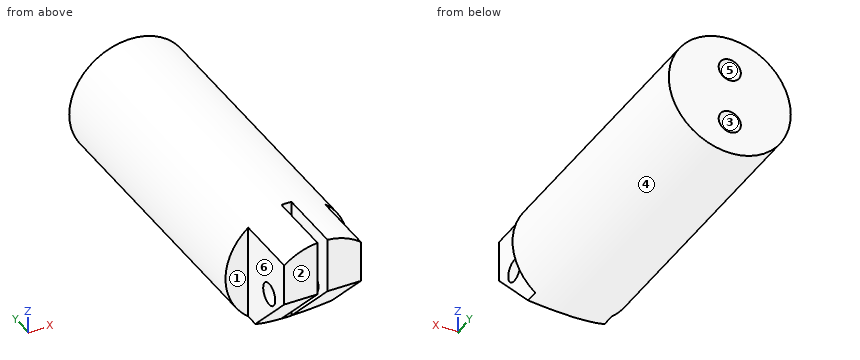
Autodesk Inventor part; units mm, degrees
ref_plane "YZ Plane" through (0, 0, 0) normal (1, 0, 0) x (0, 1, 0)
ref_plane "XZ Plane" through (0, 0, 0) normal (0, 1, 0) x (-1, 0, 0)
ref_plane "XY Plane" through (0, 0, 0) normal (0, 0, 1) x (1, 0, 0)
sketch "Sketch1" plane through (0, 0, 0) normal (0, 1, 0) x (-1, 0, 0)
  circle A0 centre (0, 0) radius 5.5
  dimension "d0" = 11
extrude "Extrusion1" add sketch "Sketch1" along normal blind 26
sketch "Sketch6" plane through (0, 0, 0) normal (0, -1, 0) x (1, 0, 0)
  circle A0 centre (0, 0) radius 5.5
  line L0 (3.45, 0) -> (3.45, -4.2834)
  line L1 (0.45, 0) -> (0.45, -5.4816)
  line L2 (3.45, -5.4816) -> (3.45, -4.2834)
  line L3 (3.45, -5.4816) -> (0.45, -5.4816)
  line L4 (0.45, 0) -> (0.45, 5.4816)
  line L5 (3.45, 5.3243) -> (3.45, 0)
  line L6 (3.45, 5.3243) -> (0.45, 5.4816)
  line L7 (0, -5.5) -> (0, 5.5)
  line L8 (-3.45, 0) -> (-3.45, -4.2834)
  line L9 (-0.45, 0) -> (-0.45, -5.4816)
  line L10 (-3.45, -5.4816) -> (-3.45, -4.2834)
  line L11 (-3.45, -5.4816) -> (-0.45, -5.4816)
  line L12 (-0.45, 0) -> (-0.45, 5.4816)
  line L13 (-3.45, 5.3243) -> (-3.45, 0)
  line L14 (-3.45, 5.3243) -> (-0.45, 5.4816)
  point P0 (-3.45, 4.2834)
  point P1 (3.45, 4.2834)
  dimension "d20" = 3
  dimension "d21" = 3
  dimension "d22" = 0.45
  dimension "d23" = 2.05
  dimension "d24" = 2.05
extrude "Extrusion5" add sketch "Sketch6" along normal blind 6 contours A0 L5 L0 L1 L4 | L12 L9 A0 L8 L13
sketch "Sketch8" plane through (0, 0, 0) normal (1, 0, 0) x (0, 1, 0)
  line L0 (0, -5.5) -> (26, -5.5)
  line L1 (0, -5.4816) -> (-6, -5.4816)
  line L2 (0, -5.4816) -> (0, 5.4816)
  line L3 (0, -5.4816) -> (-6, 0.5184)
  line L4 (0, -5.4816) -> (8.4853, -5.4816) construction
  line L5 (-6, -5.4816) -> (-6, 5.4816)
  line L6 (-6, 0.5184) -> (-6, -5.4816)
  point P0 (0, 0)
  dimension "d27" = 135
extrude "Extrusion6" cut sketch "Sketch8" along normal through all both and the other way through all
sketch "Sketch10" plane through (0, 0, 0) normal (1, 0, 0) x (0, 1, 0)
  circle A0 centre (-3.5, 0) radius 1
  line L0 (0, -5.5) -> (26, -5.5)
  line L1 (-6, 0.5184) -> (-6, 5.4816)
  point P0 (0, 0)
  dimension "d30" = 2
  dimension "d31" = 5.5
  dimension "d32" = 2.5
extrude "Extrusion7" cut sketch "Sketch10" along normal through all both and the other way through all
sketch "Sketch11" plane through (0, 26, 0) normal (0, 1, 0) x (1, 0, 0)
  circle A0 centre (0, 2.5) radius 1
  circle A1 centre (0, -2.5) radius 1
  point P0 (0, 0)
  dimension "d35" = 2
  dimension "d36" = 2
  dimension "d37" = 2.5
  dimension "d38" = 2.5
extrude "Extrusion8" cut sketch "Sketch11" against normal blind 26
properties part number "Part4 finger(pinky)"
Check sheet for the modelled part. Datum: model origin and axes. Units: mm. Face numbers are marked on the shaded views. A direction names the side the tool comes from. Round coordinates to 2 decimals unless told otherwise and drop trailing zeros. Loops run counter-clockwise (first coordinate to the right, second up) from the corner with the lowest first, then second, coordinate; pieces in that order, holes last. Notation, with made-up numbers: (50.5, -6) - (85.5, -6) arc R20 cw to (85.5, 29) - close; hole circle Ø8 at (-17.5, -36.75). An arc over 180 degrees is marked (long way). Answer as a JSON object with one key per item and string values. Group by question number.
Q1. Sectioned sample at B-B, the plane x = 0. Enter the section's corners in (y, z).
Q2. Sectioned sample at A-A, the plane z = 0. Enter the section's corners in (x, y), plus the area to 3 significant figures.
Q3. Sectioned sample at C-C, the plane y = -3.5. Enter the section's corners in (x, z).
Q4. Set-up check for the marked faces 1, 2 and 3: record each of +Z, -Z, +X, -X, +Y, -Y from which the full face is reachable in a straight line by a thin tool's end or side.
Q5. Mould release check, pull along Z, two halves, no side actions. Record for the marked faces 4, 5 and 6: released by +Z, released by -Z, zero draft, split by the parting line, or undercut.
Q6. Sectioned sample at D-D, the plane z = 2.5. Enter the section's corners in (x, y), plus the area to 3 significant figures.
Q7. Gauge pin test, flat ends, axial feed: P1, Ø3, axis at y = -4.5, z = -1, coming from the +X side; P2, Ø1.6, axis at x = 0, z = 2.5, coming from the +Y side; P3, Ø2.5, axis at x = 5, z = 0.5, coming from the -Y side. Record the tip position at first contact, or that the pin passes through.
Q8. Scan lines: line 1 along Z through (x, y) = (0, 5); line 2 along Y through (x, z) = (2.4, 0); line 3 along X through (y, z) = (-1, -2.25). Record each from-to range of solid material in increasing order. Write a range as [from, to].
Solution:
{
 "1": {"outline": "(0, -5.5) - (26, -5.5) - (26, -3.5) - (0, -3.5) - close; (0, -1.5) - (26, -1.5) - (26, 1.5) - (0, 1.5) - close; (0, 3.5) - (26, 3.5) - (26, 5.5) - (0, 5.5) - close"},
 "2": {"outline": "(-5.5, 0) - (-3.45, 0) - (-3.45, -2.5) - (-0.45, -2.5) - (-0.45, 0) - (0.45, 0) - (0.45, -2.5) - (3.45, -2.5) - (3.45, 0) - (5.5, 0) - (5.5, 26) - (-5.5, 26) - close; (-3.45, -5.48) - (-0.45, -5.48) - (-0.45, -4.5) - (-3.45, -4.5) - close; (0.45, -5.48) - (3.45, -5.48) - (3.45, -4.5) - (0.45, -4.5) - close", "area": "307 mm²"},
 "3": {"outline": "(-3.45, -1.98) - (-0.45, -1.98) - (-0.45, -1) - (-3.45, -1) - close; (-3.45, 1) - (-0.45, 1) - (-0.45, 5.48) arc R5.5 ccw to (-3.45, 4.28) - close; (0.45, -1.98) - (3.45, -1.98) - (3.45, -1) - (0.45, -1) - close; (0.45, 1) - (3.45, 1) - (3.45, 4.28) arc R5.5 ccw to (0.45, 5.48) - close"},
 "4": {"face 1": "+Z, -Z, -X, -Y", "face 2": "+Z, -Z, +X, -X, -Y", "face 3": "+Y"},
 "5": {"face 4": "split by the parting line", "face 5": "undercut", "face 6": "zero draft"},
 "6": {"outline": "(-4.9, 0) - (-3.45, 0) - (-3.45, -6) - (-0.45, -6) - (-0.45, 0) - (-1, 0) - (-1, 26) - (-4.9, 26) - close; (0.45, -6) - (3.45, -6) - (3.45, 0) - (4.9, 0) - (4.9, 26) - (1, 26) - (1, 0) - (0.45, 0) - close", "area": "239 mm²"},
 "7": {"P1": "stops at x = 3.45", "P2": "stops at y = 0", "P3": "stops at y = 0"},
 "8": {"line 1": "z = [-5.5, -3.5], [-1.5, 1.5], [3.5, 5.5]", "line 2": "y = [-5.48, -4.5], [-2.5, 26]", "line 3": "x = [-3.45, -0.45], [0.45, 3.45]"}
}
